Check sheet for the modelled part. Datum: model origin and axes. Units: mm. Round coordinates to 2 decimals unless told otherwise and drop trailing zeros. Loops run counter-clockwise (first coordinate to the right, second up) from the corner with the lowest first, then second, coordinate; pieces in that order, holes last. Notation, with made-up numbers: M -2,-4 L 45,-4 A24 ccw 45,33 Z; hole C 84,67 d9. An arc over 180 degrees is marked long. Write item = value, one per line. Start each with the question number.
(1) Scan lines: L1, parallel to Z at x = -0.5, y = 0; L2, parallel to Z at x = -2, y = -0.5; L3, parallel to Y at x = -3, z = -1.5. Record each from-to range of solid material in increasing order. Write a range as from..to.
(2) Go/stop test with flat-tipped pins: P1, Ø5.5, axis at y = 0, z = 0, coming from the +X side; P2, Ø4, axis at x = 2.5, z = 8, coming from the +Y side. Record where each tip stops, or that it passes through.
(3) Cross-section at C-C on x = 1. Record the boundary of the cut face in (y, z), plus the area to 3 significant figures.
(4) Mould release check, pull along Y, two halves, no side actions. Record for faces 1 (the face through (-3.5, 2.3, -2.3)), 2 (the face through (2.9, -2.38, -10.74)), 3 (the face through (0, 3, 0)): pulls with the +Y half, pulls with the -Y half, needs draft (parallel to the pull), parting line crosses it, or undercut.
(5) Cross-section at A-A on y = 0. Record the boundary of the cut face in (x, z), plus the area to 3 significant figures.
from build123d import *

# Parameters (mm, degrees)
F0_R          = 11
F1_DEPTH      = 3.5
F1_DEPTH_BACK = 3.5
F2_R          = 2.5
F4_R          = 3
F5_DEPTH      = 7


with BuildPart() as f1:
    # F0 (on Right) → F1 (new body, two sides)
    with BuildSketch(Plane.YZ) as f1_sk:
        Circle(F0_R)
    extrude(amount=F1_DEPTH)
    extrude(f1_sk.sketch, amount=-F1_DEPTH_BACK)

    # F2 (on Front) → F3 (revolve, cut)
    with BuildSketch(Plane.XZ):
        with Locations((0, 12)):
            Circle(F2_R)
    revolve(axis=Axis((-5, 0, 0), (-1, 0, 0)), mode=Mode.SUBTRACT)

    # F4 (on face) → F5 (cut, through all)
    with BuildSketch(Plane(origin=(-3.5, 0, 0), x_dir=(0, -1, 0), z_dir=(-1, 0, 0))):
        Circle(F4_R)
    extrude(amount=-F5_DEPTH, mode=Mode.SUBTRACT)


solid = f1.part
Result:
q1.L1 = -9.55..-3, 3..9.55
q1.L2 = -10.49..-2.96, 2.96..10.49
q1.L3 = -10.9..-2.6, 2.6..10.9
q2.P1 = through
q2.P2 = 9.22
q3.outline = C 0,0 d19.42; hole C 0,0 d6
q3.area = 268 mm^2
q4.face_1 = needs draft
q4.face_2 = parting line crosses it
q4.face_3 = undercut
q5.outline = M -3.5,-11 L -2.29,-11 A2.5 cw 2.29,-11 L 3.5,-11 L 3.5,-3 L -3.5,-3 Z; M -3.5,3 L 3.5,3 L 3.5,11 L 2.29,11 A2.5 cw -2.29,11 L -3.5,11 Z
q5.area = 102 mm^2
